Check sheet for the modelled part. Datum: model origin and axes. Units: mm. Round coordinates to 2 decimals unless told otherwise and drop trailing zeros. Loops run counter-clockwise (first coordinate to the right, second up) from the corner with the lowest first, then second, coordinate; pieces in that order, holes last. Notation, with made-up numbers: (-20, -31.75) - (12, -31.75) arc R31 ccw to (12, -5.75) - close; hole circle Ø11 at (6.5, -12.75). An arc over 180 degrees is marked (long way). Put each result on its own line as item: value.
```python
from build123d import *

# Parameters (mm, degrees)
BOSS_EXTRUDE1_DEPTH = 3.175
SKETCH2_R           = 2.286
CUT_EXTRUDE1_DEPTH  = 4.175
SKETCH3_W           = 20.32
SKETCH3_H           = 58.42
SKETCH3_W_2         = 50.8
SKETCH3_H_2         = 13.97
SKETCH3_W_3         = 13.97
SKETCH3_H_3         = 50.8
CUT_EXTRUDE2_DEPTH  = 4.175


with BuildPart() as part:
    # Sketch1 → Boss-Extrude1 (new body)
    with BuildSketch(Plane(origin=(0, 0, 0), x_dir=(1, 0, 0), z_dir=(0, 1, 0))):
        Polygon((-62.22816, -68.31704), (-29.84616, -68.31704), (-29.84616, -100.69904), (95.63984, -100.69904), (95.63984, -68.31704), (128.02184, -68.31704), (128.02184, 57.16896), (95.63984, 57.16896), (95.63984, 89.55096), (-29.84616, 89.55096), (-29.84616, 57.16896), (-62.22816, 57.16896), align=None)
    extrude(amount=BOSS_EXTRUDE1_DEPTH)

    # Sketch2 → Cut-Extrude1 (cut, through all)
    with BuildSketch(Plane(origin=(0, 3.175, 0), x_dir=(1, 0, 0), z_dir=(0, 1, 0))):
        with Locations((-24.38516, 81.93096)):
            Circle(SKETCH2_R)
        with Locations((90.17884, 81.93096)):
            Circle(SKETCH2_R)
        with Locations((90.17884, -93.07904)):
            Circle(SKETCH2_R)
        with Locations((-24.38516, -93.07904)):
            Circle(SKETCH2_R)
    extrude(amount=-CUT_EXTRUDE1_DEPTH, mode=Mode.SUBTRACT)

    # Sketch3 → Cut-Extrude2 (cut, through all)
    with BuildSketch(Plane(origin=(0, 3.175, 0), x_dir=(1, 0, 0), z_dir=(0, 1, 0))):
        with Locations((-52.06816, -5.57404)):
            Rectangle(SKETCH3_W, SKETCH3_H)
        with Locations((32.89684, 82.56596)):
            Rectangle(SKETCH3_W_2, SKETCH3_H_2)
        with Locations((121.03684, -5.57404)):
            Rectangle(SKETCH3_W_3, SKETCH3_H_3)
        with Locations((32.89684, -93.71404)):
            Rectangle(SKETCH3_W_2, SKETCH3_H_2)
    extrude(amount=-CUT_EXTRUDE2_DEPTH, mode=Mode.SUBTRACT)


solid = part.part
```
Item 1: Section check C-C on x = 30. Enter the section's corners in (y, z) (3 decimals).
Filled sheet:
outline: (0, -75.581) - (3.175, -75.581) - (3.175, 86.729) - (0, 86.729) - close
Item 2: Section check A-A on y = 2.15. Count the separate pieces of the cut face and the enclosed holes in it, then the cut area to 3 significant figures.
Filled sheet:
separate pieces: 1
enclosed holes: 4
area: 28,600 mm²
Item 3: Release check for a two-part mould opening along X. For faces 1 (the flat face through (32, 0, 4)), 2 (the cylindrical face through (-23.33, 1.61, -79.903)) record: +X half, -X half, draft (parallel to the pull), parting line (faces both ways), or undercut.
Filled sheet:
face 1: draft
face 2: undercut
Item 4: Section check B-B on z = -11.5. Enter the section's corners in (x, y) (3 decimals).
Filled sheet:
outline: (-41.908, 0) - (114.052, 0) - (114.052, 3.175) - (-41.908, 3.175) - close
Item 5: Go/stop test with flat-tipped pins: pin 1 (1 mm diameter, centred on x = 108.5, y = 2, fed in from +Z); pin 2 (4 mm diameter, centred on x = 90.18, z = 93.08, fed in from +Y); pin 3 (5.5 mm diameter, centred on x = 90.18, z = -81.93, fed in from +Y) (3 decimals); pin 4 (1 mm diameter, centred on x = -39, y = 1, fed in from -Z). Record where each tip stops, or that it passes through.
Filled sheet:
pin 1: z = 68.32
pin 2: through
pin 3: y = 3.175
pin 4: z = -57.17
Item 6: Thickness scan on line 1 (X direction, y = 1.4, z = -81.5); line 2 (X direction, y = 1, z = 90); line 3 (Z direction, x = 119, y = 0.25). Record the ranges inside material, lowest first. Write a range as from..to.
Filled sheet:
line 1: -29.85..-26.63, -22.14..7.5, 58.3..87.93, 92.42..95.64
line 2: -29.85..7.5, 58.3..95.64
line 3: -57.17..-19.83, 30.97..68.32
